Check sheet for the modelled part. Datum: model origin and axes. Units: mm. Face numbers are marked on the shaded views. Coordinates: 2 decimals unless noted, no trailing zeros. Write each loop counter-clockwise with the first axis right and the second up, starting at its lowest first coordinate (ties: lowest second). Pieces come first, ordered by that corner, then holes. Notation, with made-up numbers: (73, 65.5) - (90, 65.5) arc R20 ccw to (90, 101.5) - close; hole circle Ø5 at (40, 60). An arc over 180 degrees is marked (long way). Write each question's results on one line, items separated by ' | '.
from build123d import *

# Parameters (mm, degrees)
F0_W = 0.5
F0_H = 1.5
F2_R = 2
F3_R = 5


# Not quite as in the source:
# - a fillet or chamfer that OpenCascade refuses, or shapes differently, is made with other operations: its cross-section is extruded or revolved along the edge and cut away or added


with BuildPart() as f1:
    # F0 (on Front) → F1 (revolve)
    with BuildSketch(Plane.XZ):
        Polygon((0, 40), (0, 0), (20, 0), (20, 10), (5.45, 15), (5.45, 32.5), (5.45, 34), (5.45, 40), align=None)
        with Locations((5.7, 33.25)):
            Rectangle(F0_W, F0_H)
    revolve(axis=Axis((0, 0, 20), (0, 0, 1)))

    # F2
    f2_edges = [f1.edges().sort_by_distance(p)[0] for p in [
        (-5.45, 0, 40),
        (-5.45, 0, 15),
    ]]
    fillet(f2_edges, radius=F2_R)

    # F3
    f3_edges = [f1.edges().sort_by_distance(p)[0] for p in [
        (-20, 0, 10),
    ]]
    fillet(f3_edges, radius=F3_R)

    # F4: fillet of radius 0.7 on 3 edges, made by hand

    # F4_s1 → F4_t2 (revolve, cut)
    with BuildSketch(Plane.XZ):
        with BuildLine():
            ThreePointArc((5.45, 32.5), (5.811248608, 32.75249038), (5.95, 33.1708203932))
            Line((5.95, 33.1708203932), (5.95, 32.5))
            Line((5.95, 32.5), (5.45, 32.5))
        make_face()
    revolve(axis=Axis((0, 0, 32.5), (0, 0, 1)), mode=Mode.SUBTRACT)

    # F4_s3 → F4_t4 (revolve, cut)
    with BuildSketch(Plane.XZ):
        with BuildLine():
            ThreePointArc((5.95, 33.3291796068), (5.811248608, 33.74750962), (5.45, 34))
            Line((5.45, 34), (5.95, 34))
            Line((5.95, 34), (5.95, 33.3291796068))
        make_face()
    revolve(axis=Axis((0, 0, 34), (0, 0, 1)), mode=Mode.SUBTRACT)


solid = f1.part
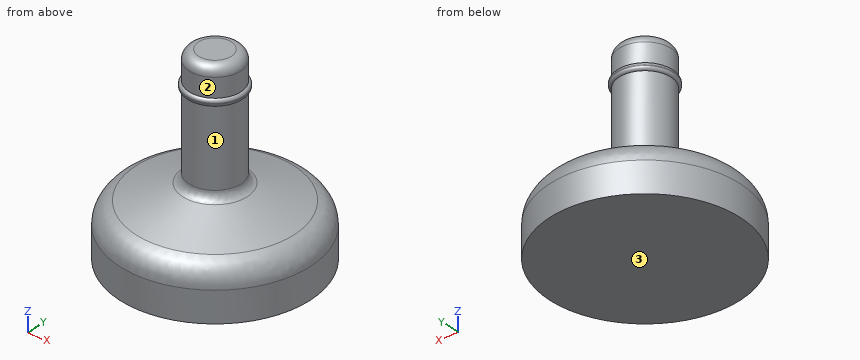
1. Draft check along Z on the marked faces 1, 2 and 3. Enter one of: pulls with the +Z half, pulls with the -Z half, needs draft (parallel to the pull), parting line crosses it, or undercut.
Values follow:
face 1: undercut | face 2: needs draft | face 3: pulls with the -Z half
2. Sectioned sample at A-A (z = 20.5). Record the cut outline in (x, y), then the cut area to 3 significant figures.
Values follow:
outline: circle Ø10.9 at (0, 0) | area: 93.3 mm^2
3. Go/stop test with flat-tipped pins: pin 1 (8 mm diameter, centred on x = -4.5, z = 34, fed in from +Y); pin 2 (4 mm diameter, centred on x = 0, z = 19, fed in from +Y); pin 3 (5 mm diameter, centred on x = 11.5, y = 4, fed in from +Z). Record where each tip stops, or that it passes through.
Values follow:
pin 1: stops at y = 5.92 | pin 2: stops at y = 5.45 | pin 3: stops at z = 13.55
4. Material ranges on L1, parallel to Z at x = -8, y = 15.5; L2, parallel to Z at x = 14, y = -8.5; L3, parallel to Y at x = -3, z = 15.5, recorded low to high. Write a range as [from, to].
Values follow:
L1: z = [0, 10.79] | L2: z = [0, 11.24] | L3: y = [-4.82, 4.82]
